Source: CAD feature listing. Evaluate the final solid. Frame: model axes, mm. Face numbers are marked on the shaded views. A direction names the side the tool comes from. Coordinates: 2 decimals unless noted, no trailing zeros. Order: outer loops, then holes, each group sorted by start corner. A loop starts at its lowest first (then second) coordinate and runs counter-clockwise, first axis right, second up.
Item 1: Mould query, pull axis X, two halves, no side actions, for the marked faces 3, 4, 5 and 6. Classes: released by +X, released by -X, zero draft, split by the parting line, or undercut.
Item 2: Section A-A on z = -50.5. Return the cut outline in (x, y), then the cut area to 3 significant figures.
Item 3: Contact query for flat-ended pins moving along their axis: P1, Ø12, axis at x = -169, z = -13, coming from the -Y side; P2, Ø12, axis at y = 89.5, z = -36, coming from the -X side; P3, Ø3, axis at y = -49, z = -15, coming from the +X side. Output: stop coordinate, or through.
Item 4: Reachability of the marked faces 1 and 2 from +Z, -Z, +X, -X, +Y, -Y: full face, straight path, thin tool, end or side. Return the list, or none.
Item 5: Ray query, line 1 (Z direction, x = -80.5, y = 31); line 2 (Y direction, x = -141.5, z = -45.5); line 3 (Y direction, x = -142, z = -44.5). Return the intervals inside material, ascending.
Item 6: Section C-C on x = -27. Return the cut outline in (y, z), then the cut area to 3 significant figures.
Item 7: Section B-B on y = -46. Return the cut outline in (x, z) (3 decimals), then the cut area to 3 significant figures.
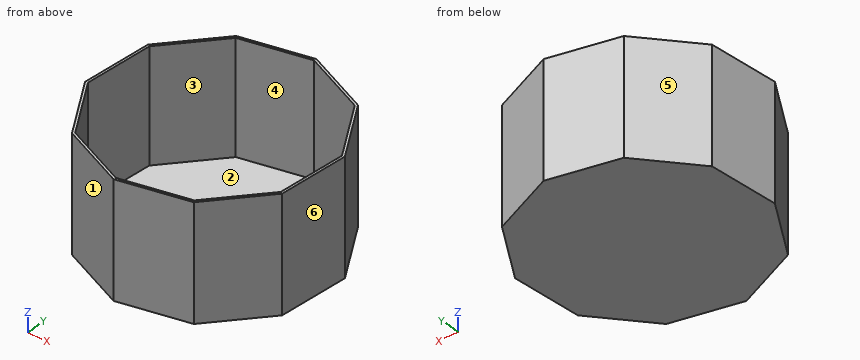
from build123d import *

# Parameters (mm, degrees)
F1_DEPTH = 122.682
F2_T     = -2.54


with BuildPart() as f1:
    # F0 (on Top) → F1 (new body)
    with BuildSketch(Plane.XY):
        Polygon((-38.383844, -96.835967), (10.351066, -41.644384), (17.337637, 31.652206), (-20.092763, 95.056997), (-87.642993, 124.351513), (-159.511162, 108.346245), (-208.246071, 53.154662), (-215.232642, -20.141928), (-177.802243, -83.546719), (-110.252012, -112.841235), align=None)
    extrude(amount=-F1_DEPTH)

    # F2
    f2_openings = [f1.faces().sort_by_distance(p)[0] for p in [
        (-98.947503, 5.755139, 0),
    ]]
    offset(amount=F2_T, openings=f2_openings)


solid = f1.part
Answer list:
1. face 3: undercut
1. face 4: undercut
1. face 5: released by -X
1. face 6: released by +X
2. outline: (-215.23, -20.14) - (-177.8, -83.55) - (-110.25, -112.84) - (-38.38, -96.84) - (10.35, -41.64) - (17.34, 31.65) - (-20.09, 95.06) - (-87.64, 124.35) - (-159.51, 108.35) - (-208.25, 53.15) - close; hole (-212.63, -19.56) - (-176.03, -81.54) - (-110, -110.18) - (-39.74, -94.54) - (7.9, -40.58) - (14.73, 31.07) - (-21.86, 93.06) - (-87.9, 121.69) - (-158.15, 106.05) - (-205.8, 52.09) - close
2. area: 1,850 mm2
3. P1: stops at y = -89.97
3. P2: stops at x = -181.45
3. P3: stops at x = 5.18
4. face 1: +Z, -Z, -X, -Y
4. face 2: +Z
5. line 1: z = -122.68 to -120.14
5. line 2: y = -99.29 to -96.52, 109.76 to 112.36
5. line 3: y = -99.07 to -96.3, 109.64 to 112.25
6. outline: (-83.94, -122.68) - (98.05, -122.68) - (98.05, 0) - (95.28, 0) - (95.28, -120.14) - (-80.11, -120.14) - (-80.11, 0) - (-83.94, 0) - close
6. area: 1,260 mm2
7. outline: (-199.968, -122.682) - (6.505, -122.682) - (6.505, 0) - (3.116, 0) - (3.116, -120.142) - (-197.018, -120.142) - (-197.018, 0) - (-199.968, 0) - close
7. area: 1,290 mm2
